from build123d import *

# Parameters (mm, degrees)
SKETCH2_R          = 2
CUT_EXTRUDE2_DEPTH = 18
SKETCH3_R          = 4.5
CUT_EXTRUDE3_DEPTH = 2
CHAMFER2_SIZE      = 3


with BuildPart() as part:
    # Sketch1 → Revolve1 (revolve)
    with BuildSketch(Plane(origin=(0, 0, 0), x_dir=(1, 0, 0), z_dir=(0, 1, 0)), mode=Mode.PRIVATE) as revolve1_sk:
        Polygon((-30.147058824, 0), (-30.147058824, 10), (-25.147058824, 10), (-19.705882353, 6.176470588), (-10.147058824, 6.176470588), (-10.147058824, 0), align=None)
    revolve(revolve1_sk.sketch.rotate(Axis((-68.088235294, 0, 0), (1, 0, 0)), 180), axis=Axis((-68.088235294, 0, 0), (1, 0, 0)))

    # Sketch2 → Cut-Extrude2 (cut)
    with BuildSketch(Plane(origin=(-10.147058824, 0, 0), x_dir=(0, 0, -1), z_dir=(1, 0, 0))):
        Circle(SKETCH2_R)
    extrude(amount=-CUT_EXTRUDE2_DEPTH, mode=Mode.SUBTRACT)

    # Sketch3 → Cut-Extrude3 (cut)
    with BuildSketch(Plane.ZY.offset(30.147058824)):
        Circle(SKETCH3_R)
    extrude(amount=-CUT_EXTRUDE3_DEPTH, mode=Mode.SUBTRACT)

    # Chamfer2
    # the kernel refuses this chamfer: 3 mm, written as the material it takes off along each edge
    with BuildSketch(Plane(origin=(-28.147058824, 0, 0), x_dir=(0, 0, -1), z_dir=(0, -1, 0))) as chamfer2_piece_1_section:
        Polygon((2 + CHAMFER2_SIZE, 0), (2, CHAMFER2_SIZE), (2, 0), align=None)
    chamfer2_piece_1 = revolve(axis=Axis((-28.147058824, 0, 0), (1, 0, 0)), mode=Mode.PRIVATE)
    chamfer2_piece_1 = chamfer2_piece_1 & Plane(origin=(-26.385999782, 0, 0), x_dir=(0, 0, 1), z_dir=(-1, 0, 0)) * Cylinder(4.5, 20, mode=Mode.PRIVATE)
    add(chamfer2_piece_1, mode=Mode.SUBTRACT)


solid = part.part
Can you work these out from the model? Positions are in its coordinate system, mm. A direction names the side the tool comes from. Round coordinates to 2 decimals unless told otherwise and drop trailing zeros. Write each loop counter-clockwise with the first axis right and the second up, starting at its lowest first coordinate (ties: lowest second). Pieces come first, ordered by that corner, then holes. Notation, with made-up numbers: (16.25, 51) - (51.25, 51) arc R10 ccw to (51.25, 60) - close; hole circle Ø7 at (69.5, 74). An arc over 180 degrees is marked (long way). Write each question's results on one line, items separated by ' | '. Start each with the question number.
1) Suppose I cut it at C-C (x = -13). List the corners of the cut face in (y, z) for me, and give its area (3 significant figures).
2) Suppose I cut it at D-D (x = -23.5). List the corners of the cut face in (y, z) for me, and give its area (3 significant figures).
3) Please list where these lines run through material, in increasing order: line 1 (Y direction, x = -28.85, z = 0); line 2 (Y direction, x = -16.5, z = 0); line 3 (Z direction, x = -29, y = -3.25).
4) We'd pull the mould along Y, two halves only. Please class faces 3 (the cylindrical face through (-28.915, 1.352, 4.292)), 4 (the flat face through (-10.147, 0, 3)), 5 (the conical face through (-19.97, 6.21, -1.38)): released by +Y, released by -Y, zero draft, split by the parting line, or undercut.
5) Suppose I cut it at A-A (z = 0). List the corners of the cut face in (x, y) for me.
6) Which directions (+Z, -Z, +X, -X, +Y, -Y) give clear straight access to the entire face, cutting with the end or side of a thin tool? Please do faces 1 (the cylindrical face through (-28, 0, -10)), 2 (the cylindrical face through (-14.86, -6.124, -0.804)).
7) For pin 1 Ø6 at (x, z) = (-16.5, 2.5) entering from +Y; pin 2 Ø8 at (x, y) = (-14, 3.5) entering from -Z; pin 3 Ø6 at (x, z) = (-17.5, -0.5) entering from -Y; pin 4 Ø12 at (y, z) = (-1, -3.5) entering from -X, each with a flat end and sliding along its axis, tell me the tip position at first contact or that it passes through.
Here are the results:
1) outline: circle Ø12.35 at (0, 0); hole circle Ø4 at (0, 0) | area: 107 mm2
2) outline: circle Ø17.69 at (0, 0); hole circle Ø4 at (0, 0) | area: 233 mm2
3) line 1: y = -10 to -4.5, 4.5 to 10 | line 2: y = -6.18 to -2, 2 to 6.18 | line 3: z = -9.46 to -3.11, 3.11 to 9.46
4) face 3: undercut | face 4: zero draft | face 5: split by the parting line
5) outline: (-30.15, -10) - (-25.15, -10) - (-19.71, -6.18) - (-10.15, -6.18) - (-10.15, -2) - (-25.15, -2) - (-27.65, -4.5) - (-30.15, -4.5) - close; (-30.15, 4.5) - (-27.65, 4.5) - (-25.15, 2) - (-10.15, 2) - (-10.15, 6.18) - (-19.71, 6.18) - (-25.15, 10) - (-30.15, 10) - close
6) face 1: +X, -X | face 2: +X
7) pin 1: stops at y = 6.18 | pin 2: stops at z = -6.18 | pin 3: stops at y = -6.72 | pin 4: stops at x = -30.15
